Autodesk Inventor part; units mm, degrees
ref_plane "YZ Plane" through (0, 0, 0) normal (1, 0, 0) x (0, 1, 0)
ref_plane "XZ Plane" through (0, 0, 0) normal (0, 1, 0) x (-1, 0, 0)
ref_plane "XY Plane" through (0, 0, 0) normal (0, 0, 1) x (1, 0, 0)
sketch "Sketch3" plane through (0, 0, 0) normal (0, 1, 0) x (-1, 0, 0)
  line L0 (0, 0) -> (0, -60)
  line L1 (0, 0) -> (60, 0) construction
  line L2 (0, -60) -> (12.519, -60)
  line L3 (0, 0) -> (25.4, 0)
  line L4 (25.4, 0) -> (25.4, 7.5)
  arc A0 (40.4, 7.5) -> (25.4, 7.5) centre (32.9, 7.5) ccw
  line L5 (40.4, 7.5) -> (40.4, -16.519)
  line L6 (40.4, -16.519) -> (12.519, -60)
  line L7 (0, -30) -> (5, -30)
  line L8 (5, -60) -> (5, -48)
  line L9 (5, 0) -> (5, -12)
  circle A1 centre (5, -12) radius 1.5
  circle A2 centre (5, -48) radius 1.5
  circle A3 centre (32.9, 7.5) radius 4
  line L10 (32.9, 7.5) -> (32.9, -3.512)
  line L11 (32.9, -3.512) -> (32.9, -10.02)
  circle A4 centre (32.9, -3.512) radius 1
  circle A5 centre (32.9, -10.02) radius 1
  dimension "d6" = 60
  dimension "d7" = 90
  dimension "d8" = 12.519
  dimension "d9" = 25.4
  dimension "d10" = 7.5
  dimension "d11" = 15
  dimension "d13" = 24.019
  dimension "d18" = 5
  dimension "d19" = 12
  dimension "d20" = 12
  dimension "d21" = 3
  dimension "d22" = 3
  dimension "d25" = 8
  dimension "d26" = 11.012
  dimension "d27" = 6.508
  dimension "d28" = 2
  dimension "d29" = 2
extrude "Extrusion1" add sketch "Sketch3" along normal blind 3
sketch "Sketch6" plane through (0, 3, 0) normal (0, 1, 0) x (1, 0, 0)
  circle A0 centre (-32.9, -7.5) radius 4
  circle A1 centre (-5, 48) radius 1.5
  circle A2 centre (-5, 12) radius 1.5
  circle A3 centre (-32.9, 10.02) radius 1
  circle A4 centre (-32.9, 3.512) radius 1
  line L0 (0, 0) -> (0, 60)
  line L1 (0, 60) -> (-12.519, 60)
  line L2 (-12.519, 60) -> (-40.4, 16.519)
  line L3 (-40.4, 16.519) -> (-40.4, -7.5)
  arc A5 (-40.4, -7.5) -> (-25.4, -7.5) centre (-32.9, -7.5) ccw
  line L4 (-25.4, -7.5) -> (-25.4, 0)
  line L5 (-25.4, 0) -> (0, 0)
  line L6 (-40.4, 16.519) -> (-25.4, 16.519)
  line L7 (-25.4, -7.5) -> (-25.4, 0)
  line L8 (-25.4, 16.519) -> (-25.4, 0)
  circle A6 centre (-32.9, -7.5) radius 5.5
  line L9 (-32.9, 10.02) -> (-32.9, 11.52)
  circle A7 centre (-32.9, 11.52) radius 3
  line L10 (-38.4, -7.5) -> (-38.4, -4.5)
  line L11 (-27.4, -7.5) -> (-27.4, -4.5)
  line L12 (-27.4, -4.5) -> (-29.9349, 11.9762)
  line L13 (-38.4, -4.5) -> (-35.8651, 11.9762)
  point P0 (0, 0)
  dimension "d31" = 11
  dimension "d32" = 1.5
  dimension "d33" = 6
  dimension "d34" = 3
extrude "Extrusion3" add sketch "Sketch6" against normal blind 6 contours L4 A5 L3 L6 L8
properties part number "servoSideShort"
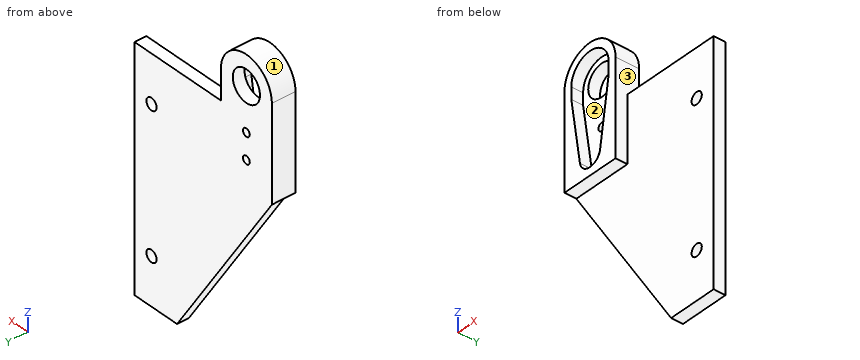
The listing builds one solid part. Answer for the finished solid, in the listing's coordinates (mm). Face numbers are marked on the shaded views. Round coordinates to 2 decimals unless told otherwise and drop trailing zeros. Order: outer loops, then holes, each group sorted by start corner. A loop starts at its lowest first (then second) coordinate and runs counter-clockwise, first axis right, second up. Notation, with made-up numbers: (-35.5, 80.5) - (19.5, 80.5) arc R7 ccw to (19.5, 85.5) - close; hole circle Ø4 at (22.25, 61). An arc over 180 degrees is marked (long way). Put each result on its own line as item: value. Start each with the question number.
(1) Find section C-C (y = -1). Give the vertices of the cut face in (x, z), plus the area to 3 significant figures.
(2) Find section A-A (z = 9.5). Give the vertices of the cut face in (x, y), plus the area to 3 significant figures.
(3) Straight lines are drawn through the part: probe 1 along X at (y, z) = (-0.35, 5); probe 2 along X at (y, z) = (2.1, -12); probe 3 along X at (y, z) = (2.6, 1). For each, find the intervals that lie inside material, in ascending order. Write a range as from..to.
(4) Determine the mould class of the marked faces 1, 2 and 3 for opening direction Z: released by +Z, released by -Z, zero draft, split by the parting line, or undercut.
(5) Find section B-B (x = -5). Give the vertices of the cut face in (y, z), plus the area to 3 significant figures.
(6) Given P1, Ø3, axis at x = -15.5, z = -14, coming from the -Y side; P2, Ø2.5, axis at y = -1, z = 6.5, coming from the +X side; P3, Ø3.5, axis at x = -9, y = 2, coming from the +Z side, each flat-ended and moving along its own axis, determine where each tip first touches the part or whether it passes through.
(7) Find section D-D (x = -32.9). Give the vertices of the cut face in (y, z), plus the area to 3 significant figures.
Reply:
1. outline: (-40.4, -16.52) - (-25.4, -16.52) - (-25.4, 7.5) arc R7.5 ccw to (-40.4, 7.5) - close; hole (-38.4, 4.5) - (-35.87, -11.98) arc R3 ccw to (-29.93, -11.98) - (-27.4, 4.5) - (-27.4, 7.5) arc R5.5 ccw to (-38.4, 7.5) - close
1. area: 217 mm^2
2. outline: (-40.13, -3) - (-38.02, -3) - (-38.02, 0) - (-36.36, 0) - (-36.36, 3) - (-40.13, 3) - close; (-29.44, 0) - (-27.78, 0) - (-27.78, -3) - (-25.67, -3) - (-25.67, 3) - (-29.44, 3) - close
2. area: 35.2 mm^2
3. probe 1: -40.4..-38.4, -27.4..-25.4
3. probe 2: -40.4..-6.5, -3.5..0
3. probe 3: -40.4..-25.4
4. face 1: released by +Z
4. face 2: undercut
4. face 3: zero draft
5. outline: (0, -60) - (3, -60) - (3, -49.5) - (0, -49.5) - close; (0, -46.5) - (3, -46.5) - (3, -13.5) - (0, -13.5) - close; (0, -10.5) - (3, -10.5) - (3, 0) - (0, 0) - close
5. area: 162 mm^2
6. P1: y = 0
6. P2: x = -25.4
6. P3: z = 0
7. outline: (-3, -16.52) - (0, -16.52) - (0, -28.22) - (3, -28.22) - (3, -11.02) - (0, -11.02) - (0, -14.52) - (-3, -14.52) - close; (-3, 13) - (0, 13) - (0, 11.5) - (3, 11.5) - (3, 15) - (-3, 15) - close; (0, -9.02) - (3, -9.02) - (3, -4.51) - (0, -4.51) - close; (0, -2.51) - (3, -2.51) - (3, 3.5) - (0, 3.5) - close
7. area: 106 mm^2
